Read the model definition and answer for the solid it produces. Units are mm, in the model's axes. A direction names the side the tool comes from. Round coordinates to 2 decimals unless told otherwise and drop trailing zeros. Loops run counter-clockwise (first coordinate to the right, second up) from the corner with the lowest first, then second, coordinate; pieces in that order, holes last. Notation, with made-up numbers: (4.5, 69) -> (24.5, 69) arc R18 cw to (24.5, 97) -> close; hole circle Ø3 at (61.5, -33). An arc over 180 degrees is marked (long way). Put each result on its own line as item: value.
from build123d import *
from build123d.topology import SkipClean

# Parameters (mm, degrees)
SKETCH1_R           = 14
BOSS_EXTRUDE1_DEPTH = 19
BOSS_EXTRUDE2_DEPTH = 1
CUT_EXTRUDE1_REACH  = 33.591
SKETCH3_R           = 2.1
BOSS_EXTRUDE3_DEPTH = 16
SKETCH5_R           = 4.5
BOSS_EXTRUDE4_DEPTH = 1.5
SKETCH6_R           = 2.5
BOSS_EXTRUDE5_DEPTH = 2.5
BOSS_EXTRUDE6_DEPTH = 6


with BuildPart() as part:
    # Sketch1 → Boss-Extrude1 (new body)
    with BuildSketch(Plane(origin=(0, 0, 0), x_dir=(1, 0, 0), z_dir=(0, 1, 0))):
        with Locations(Location((0, 0, 0), (0, 0, 270))):
            Circle(SKETCH1_R)
    extrude(amount=BOSS_EXTRUDE1_DEPTH)

    # Sketch2 → Boss-Extrude2 (add)
    with BuildSketch(Plane(origin=(0, 19, 0), x_dir=(1, 0, 0), z_dir=(0, 1, 0))):
        with BuildLine():
            Line((13.555441712, 3.5), (17.5, 3.5))
            ThreePointArc((17.5, 3.5), (21, 0), (17.5, -3.5))
            Line((17.5, -3.5), (13.555441712, -3.5))
            ThreePointArc((13.555441712, -3.5), (14, 0), (13.555441712, 3.5))
        make_face()
        with BuildLine():
            Line((-13.555441712, -3.5), (-17.5, -3.5))
            ThreePointArc((-17.5, -3.5), (-21, 0), (-17.5, 3.5))
            Line((-17.5, 3.5), (-13.555441712, 3.5))
            ThreePointArc((-13.555441712, 3.5), (-14, 0), (-13.555441712, -3.5))
        make_face()
    extrude(amount=-BOSS_EXTRUDE2_DEPTH)

    # Sketch3 → Cut-Extrude1 (cut, up to next)
    with BuildSketch(Plane(origin=(0, 19, 0), x_dir=(1, 0, 0), z_dir=(0, 1, 0)), mode=Mode.PRIVATE) as cut_extrude1_sk1:
        with Locations(Location((17.5, 0, 0), (0, 0, 270))):
            Circle(SKETCH3_R)
    cut_extrude1_tool1 = extrude(cut_extrude1_sk1.sketch, amount=-CUT_EXTRUDE1_REACH, mode=Mode.PRIVATE) & part.part
    # Sketch3 → Cut-Extrude1 (cut, up to next)
    with BuildSketch(Plane(origin=(0, 19, 0), x_dir=(1, 0, 0), z_dir=(0, 1, 0)), mode=Mode.PRIVATE) as cut_extrude1_sk2:
        with Locations(Location((-17.5, 0, 0), (0, 0, 270))):
            Circle(SKETCH3_R)
    cut_extrude1_tool2 = extrude(cut_extrude1_sk2.sketch, amount=-CUT_EXTRUDE1_REACH, mode=Mode.PRIVATE) & part.part
    add(cut_extrude1_tool1.solids().sort_by_distance((17.5, 19, 0))[0], mode=Mode.SUBTRACT)
    add(cut_extrude1_tool2.solids().sort_by_distance((-17.5, 19, 0))[0], mode=Mode.SUBTRACT)

    # Sketch4 → Boss-Extrude3 (add)
    with BuildSketch(Plane(origin=(0, 19, 0), x_dir=(1, 0, 0), z_dir=(0, 1, 0))):
        with BuildLine():
            Line((7.3, -11.94612908), (7.3, -17))
            Line((7.3, -17), (-7.3, -17))
            Line((-7.3, -17), (-7.3, -11.94612908))
            ThreePointArc((-7.3, -11.94612908), (0, -14), (7.3, -11.94612908))
        make_face()
    extrude(amount=-BOSS_EXTRUDE3_DEPTH)

    # Sketch5 → Boss-Extrude4 (add)
    with BuildSketch(Plane(origin=(0, 19, 0), x_dir=(1, 0, 0), z_dir=(0, 1, 0))):
        with Locations(Location((0, 8, 0), (0, 0, 270))):
            Circle(SKETCH5_R)
    extrude(amount=BOSS_EXTRUDE4_DEPTH)

    # Sketch6 → Boss-Extrude5 (add)
    with BuildSketch(Plane(origin=(0, 20.5, 0), x_dir=(1, 0, 0), z_dir=(0, 1, 0))):
        with Locations(Location((0, 8, 0), (0, 0, 270))):
            Circle(SKETCH6_R)
    extrude(amount=BOSS_EXTRUDE5_DEPTH)

    # Sketch7 → Boss-Extrude6 (add)
    with SkipClean():  # the faces are left unmerged after this step: merging them gives an invalid solid
        with BuildSketch(Plane(origin=(0, 23, 0), x_dir=(1, 0, 0), z_dir=(0, 1, 0))):
            with BuildLine():
                Line((-2, 9.5), (2, 9.5))
                ThreePointArc((2, 9.5), (2.5, 8), (2, 6.5))
                Line((2, 6.5), (-2, 6.5))
                ThreePointArc((-2, 6.5), (-2.5, 8), (-2, 9.5))
            make_face()
        extrude(amount=BOSS_EXTRUDE6_DEPTH)


solid = part.part
Item 1: The part is cut by section D-D (y = 25.25). Determine the outline of the cut face in (x, z).
Derived:
outline: (-2, -9.5) -> (2, -9.5) arc R2.5 ccw to (2, -6.5) -> (-2, -6.5) arc R2.5 ccw to start
Item 2: Which of the six approach directions +Z, -Z, +X, -X, +Y, -Y give full straight-line access (tool end or side, diameter ignored) to faces 1 (the cylindrical face through (0.616, 9.367, -13.986)), 2 (the flat face through (15.5, 18.5, -3.5)), 3 (the flat face through (0, 26, -6.5)), 4 (the flat face through (-15.5, 18.5, 3.5)), 5 (the flat face through (7.3, 11, 14))?
Derived:
face 1: -Y
face 2: -Z, +X, +Y, -Y
face 3: +Z, +X, -X, +Y
face 4: +Z, -X, +Y, -Y
face 5: +Z, +X, +Y, -Y
Item 3: The part is cut by section A-A (z = 0). Determine the outline of the cut face in (x, y), then the cut area to 3 significant figures.
Derived:
outline: (-21, 18) -> (-19.6, 18) -> (-19.6, 19) -> (-21, 19) -> close; (-15.4, 18) -> (-14, 18) -> (-14, 0) -> (14, 0) -> (14, 18) -> (15.4, 18) -> (15.4, 19) -> (-15.4, 19) -> close; (19.6, 18) -> (21, 18) -> (21, 19) -> (19.6, 19) -> close
area: 538 mm^2
Item 4: The part is cut by section B-B (x = 17). Determine the outline of the cut face in (y, z).
Derived:
outline: (18, -3.5) -> (19, -3.5) -> (19, -2.04) -> (18, -2.04) -> close; (18, 2.04) -> (19, 2.04) -> (19, 3.5) -> (18, 3.5) -> close
Item 5: Flat-ended cylindrical pins translate along their axes: pin 1 Ø4.5 at (x, y) = (0, 27) entering from -Z; pin 2 Ø8 at (x, z) = (-13, 5) entering from +Y; pin 3 Ø3.5 at (x, z) = (-17.5, 0) entering from -Y; pin 4 Ø3 at (x, y) = (0, 27) entering from +Z. Find the tip coordinate at first contact, or state that the pin passes through.
Derived:
pin 1: stops at z = -9.5
pin 2: stops at y = 19
pin 3: passes through
pin 4: stops at z = -6.5
Item 6: Find the intervals of material crossed by line 1 along X through (y, z) = (18.85, 0); line 2 along Y through (x, z) = (-11.5, 5.5); line 3 along Y through (x, z) = (-3, -10.5), in increasing order.
Derived:
line 1: x = -21 to -19.6, -15.4 to 15.4, 19.6 to 21
line 2: y = 0 to 19
line 3: y = 0 to 20.5
Item 7: For a pull along X with two mould halves and no side action, classify faces 6 (the cylindrical face through (-21, 18.5, 0.1)), 7 (the flat face through (-15.6, 18.5, -3.5)), 8 (the cylindrical face through (-15.418, 18.507, -0.273)) as pulls with the +X half, pulls with the -X half, needs draft (parallel to the pull), parting line crosses it, or undercut.
Derived:
face 6: pulls with the -X half
face 7: needs draft
face 8: undercut
Item 8: The part is cut by section C-C (z = 13). Determine the outline of the cut face in (x, y).
Derived:
outline: (-7.3, 3) -> (-5.2, 3) -> (-5.2, 0) -> (5.2, 0) -> (5.2, 3) -> (7.3, 3) -> (7.3, 19) -> (-7.3, 19) -> close
